Check sheet for the modelled part. Datum: model origin and axes. Units: mm. A direction names the side the tool comes from. Round coordinates to 2 decimals unless told otherwise and drop trailing zeros. Loops run counter-clockwise (first coordinate to the right, second up) from the corner with the lowest first, then second, coordinate; pieces in that order, holes last. Notation, with made-up numbers: (53.25, -33) - (77.25, -33) arc R31 cw to (77.25, -6) - close; hole circle Ø4 at (40.5, -39). An arc over 180 degrees is marked (long way). Answer in a Markdown table with one row per item. Add a question column.
(1) Thickness scan on line 1 along X through (y, z) = (-0.1, -0.7); line 2 along Y through (x, z) = (0.5, -0.5); line 3 along X through (y, z) = (0.95, 1.45). Record the ranges inside material, lowest first.
(2) Cross-section at A-A on y = 0. Enter the section's corners in (x, z).
(3) Cross-section at B-B on z = 0. Enter the section's corners in (x, y), then the cut area to 3 significant figures.
(4) Gauge pin test, flat ends, axial feed: pin 1 (1 mm diameter, centred on x = 4.5, y = 0.5, fed in from +Z); pin 2 (0.5 mm diameter, centred on x = 0.5, z = 0.5, fed in from -Y); pin 3 (1 mm diameter, centred on x = 5, z = -0.5, fed in from +Y). Record the tip position at first contact, or that the pin passes through.
(5) Access from +Z, -Z, +X, -X, +Y, -Y to the whole of each face (thin tool, end or side, straight path). Record for faces 4 (the cylindrical face through (0.15, 1.9, 0.04)), 5 (the flat face through (0.4, 0.15, 0)).
(6) Mould release check, pull along Y, two halves, no side actions. Record for faces 1 (the cylindrical face through (4, 0, 1)), 2 (the flat face through (0.4, -0.15, 0)), 3 (the cylindrical face through (0.15, -1.9, -0.04)): +Y half, -Y half, draft (parallel to the pull), parting line (faces both ways), or undercut.
(7) Cross-section at D-D on x = 5. Enter the section's corners in (y, z), then the cut area to 3 significant figures.
Autodesk Inventor part; units mm, degrees
ref_plane "Work Plane1" through (33.575, 0, 0) normal (0, 0, -1) x (1, 0, 0)
ref_plane "YZ Plane" through (0, 0, 0) normal (1, 0, 0) x (0, 1, 0)
ref_plane "XZ Plane" through (0, 0, 0) normal (0, 1, 0) x (-1, 0, 0)
sketch "Эскиз1" plane through (0, 0, 0) normal (0, 0, 1) x (1, 0, 0)
  line L0 (0, 0) -> (6, 0)
  line L1 (6, 0) -> (6, 1)
  line L2 (6, 1) -> (1.6, 1)
  line L3 (1.6, 1) -> (1.3546, 1)
  line L4 (1.3546, 1) -> (1.2, 1)
  line L5 (1.2, 1) -> (0.3, 1.9)
  line L6 (0.3, 1.9) -> (0, 1.9)
  line L7 (0, 1.9) -> (0, 0)
  line L8 (1.6, 1) -> (1.2, 1) construction
  line L9 (-1.2, 0) -> (7.2, 0)
  line L10 (0, 2.28) -> (0, -0.38)
  dimension "d0" = 6
  dimension "d1" = 45
  dimension "d2" = 0.2454
  dimension "d3" = 4.4
  dimension "d4" = 1.2
  dimension "d5" = 2
  dimension "d6" = 2
  dimension "d7" = 3.8
revolve "Базовый элемент" add sketch "Эскиз1" angle 360 about axis through (0, 0, 0) along (1, 0, 0)
sketch "Эскиз2" plane through (0, 0, 0) normal (-1, 0, 0) x (0, 0, 1)
  line L0 (1.9, -0.15) -> (-1.9, -0.15)
  line L1 (-1.9, -0.15) -> (-1.9, 0.15)
  line L2 (-1.9, 0.15) -> (1.9, 0.15)
  line L3 (1.9, 0.15) -> (1.9, -0.15)
  line L4 (0, 0.15) -> (0, -0.15) construction
  line L5 (-1.9, 0) -> (1.9, 0) construction
  line L6 (0, 1.9) -> (0, 0)
  dimension "d15" = 0.3
  dimension "d16" = 3.8
extrude "Паз" cut sketch "Эскиз2" against normal blind 0.9
thread "Резьба"
chamfer "Фаска1" distance 0.2454 distance2 0.1227 1 edges at (6, -1, 0) measured on face at (6, -0.0858, 0.7069)
ref_plane "Work Plane1" through (33.575, 0, 0) normal (0, 0, -1) x (1, 0, 0)
equation "\"d0\" = NLG"
equation "\"d1\" = 0.5 * SEWI"
equation "\"d2\" = GAL"
equation "\"d3\" = GEL"
equation "\"d4\" = KOH"
equation "\"d5\" = BDM"
equation "\"d6\" = GD"
equation "\"d7\" = KOD"
equation "\"d15\" = SBR"
equation "\"d16\" = KOD"
equation "\"d8\" = STI"
equation "\"d10\" = GEL"
equation "\"d12\" = -0.5 * SPD + 0.5 * GD"
equation "\"d13\" = 0.5 * GAL"
equation "\"NLG\" = 6"
equation "\"GAL\" = 0.61345 * PTC"
equation "\"GEL\" = 4.4"
equation "\"KOH\" = 1.2"
equation "\"KOD\" = 3.8"
equation "\"SEWI\" = 90deg"
equation "\"BDM\" = NND"
equation "\"GD\" = NND"
equation "\"SBR\" = 0.3"
equation "\"STI\" = 0.9"
equation "\"SPD\" = NND - 1.2269 * PTC"
equation "\"GUL\" = 0.61345 * PTC"
equation "\"PTC\" = 0.4"
equation "\"EPV\" = 2.2"
equation "\"THREADDIA\" = 2"
equation "\"TOA\" = 30deg"
equation "\"FAWI\" = 45deg"
equation "\"RR\" = 0.1 * NND"
equation "\"NND\" = 2"
equation "\"GD1\" = THREADDIA - 1.2269 * PTC"
properties part number "Винт M2-6gx6 ГОСТ 17475-80" material "Сталь, мягкая"
Answers:
| question | item | result |
|---|---|---|
| 1 | line 1 | x = 0.9 to 6 |
| 1 | line 2 | y = -1.62 to -0.15, 0.15 to 1.62 |
| 1 | line 3 | x = 0 to 0.47 |
| 2 | outline | (0.9, -1.3) - (1.2, -1) - (5.88, -1) - (6, -0.75) - (6, 0.75) - (5.88, 1) - (1.2, 1) - (0.9, 1.3) - close |
| 3 | outline | (0, -1.9) - (0.3, -1.9) - (1.2, -1) - (5.88, -1) - (6, -0.75) - (6, 0.75) - (5.88, 1) - (1.2, 1) - (0.3, 1.9) - (0, 1.9) - (0, 0.15) - (0.9, 0.15) - (0.9, -0.15) - (0, -0.15) - close |
| 3 | area | 13.0 mm^2 |
| 4 | pin 1 | stops at z = 1 |
| 4 | pin 2 | stops at y = -1.87 |
| 4 | pin 3 | stops at y = 1 |
| 5 | face 4 | +X, -X, +Y |
| 5 | face 5 | +Z, -Z, -X |
| 6 | face 1 | parting line |
| 6 | face 2 | undercut |
| 6 | face 3 | -Y half |
| 7 | outline | circle Ø2 at (0, 0) |
| 7 | area | 3.14 mm^2 |
